The model under review builds one solid part; all positions refer to its coordinate system, in mm. A direction names the side the tool comes from. Round coordinates to 2 decimals unless told otherwise and drop trailing zeros. Loops run counter-clockwise (first coordinate to the right, second up) from the corner with the lowest first, then second, coordinate; pieces in that order, holes last. Notation, with made-up numbers: M 65,-32 L 83,-32 A15 cw 83,-9 Z; hole C 71,-15.75 d10. An arc over 180 degrees is marked long. Answer as a JSON object with one key per item and string values. Group by question number.
Item 1: To check wall thickness, follow line 1 (Z direction, x = -9, y = 0.3); line 2 (Z direction, x = -87.5, y = 3.35); line 3 (Z direction, x = 0, y = 4.6). State the ranges of each line that lie inside material, in increasing order.
Item 2: Insertion check: P1, Ø8, axis at x = -88.58, z = -718, coming from the +Y side; P2, Ø5.5, axis at x = -30.98, z = -734, coming from the -Y side; P3, Ø1, axis at y = 1, z = 82, coming from the +X side; P4, Ø3, axis at y = 3, z = 297.5, coming from the +X side. Each pin has a flat end and moves straight along its axis. Give the tip position at first contact, or say it passes through.
Item 3: The part is to be moulded in two halves that separate along Z. For faces 1 (the face through (-181, 0, 10)), 2 (the face through (85.906, 2.465, 451.968)), 3 (the face through (-249.98, 2.46, 10.62)), say which applies: +Z half, -Z half, draft (parallel to the pull), parting line (faces both ways), or undercut.
Item 4: Tool access review of faces 4 (the face through (84.55, 2.46, -443.41)), 5 (the face through (-149.945, 2.535, -4.063)): name each direction out of +Z, -Z, +X, -X, +Y, -Y from which nothing blocks a thin tool from reaching the whole face with its end or side.
Item 5: Consider section C-C (x = -105.5). Give the boundary of the cut face in (y, z).
Item 6: Consider section B-B (y = 1.8). State how many separate pieces and enclosed holes the cut face has, and give its area (3 significant figures).
Item 7: Consider section D-D (z = 0). Give the boundary of the cut face in (x, y), and give its area (3 significant figures).
Item 8: Consider section A-A (x = 0). Give the boundary of the cut face in (y, z).
Autodesk Inventor part; units mm, degrees
ref_plane "YZ Plane" through (0, 0, 0) normal (1, 0, 0) x (0, 1, 0)
ref_plane "XZ Plane" through (0, 0, 0) normal (0, 1, 0) x (-1, 0, 0)
ref_plane "XY Plane" through (0, 0, 0) normal (0, 0, 1) x (1, 0, 0)
sketch "Sketch1" plane through (0, 0, 0) normal (0, 1, 0) x (-1, 0, 0)
  arc A0 (0, -750) -> (0, 750) centre (-2762.5, 0) ccw construction
  line L0 (-22.4292, 0) -> (36.1533, 0) construction
  line L1 (0, 750) -> (0, -750) construction
  line L2 (150, 750) -> (-150, 750)
  line L3 (150, -750) -> (-150, -750)
  arc A1 (150, -750) -> (150, 750) centre (-2612.5, 0) ccw
  arc A2 (-150, -750) -> (-150, 750) centre (-2912.5, 0) ccw
  point P0 (0, 0)
  point P1 (100, 0)
  point P2 (250, 0)
  point P3 (-50, 0)
  dimension "d0" = 1500
  dimension "d1" = 100
  dimension "d2" = 300
  dimension "d3" = 150
  dimension "d4" = 150
extrude "Extrusion1" add sketch "Sketch1" along normal blind 5
sketch "Sketch2" plane through (0, 5, 0) normal (0, 1, 0) x (1, 0, 0)
  line L0 (-150, -750) -> (150, -750) construction
  arc A0 (150, 750) -> (150, -750) centre (2912.5, 0) ccw construction
  line L1 (150, 750) -> (-150, 750) construction
  arc A1 (-150, 750) -> (-150, -750) centre (2612.5, 0) ccw construction
  line L2 (-150, -750) -> (150, -750) construction
  arc A2 (150, 750) -> (150, -750) centre (2912.5, 0) ccw construction
  line L3 (150, -750) -> (150, -750) construction
  line L4 (150, -750) -> (150, -750) construction
  line L5 (150, 750) -> (-150, 750) construction
  line L6 (150, -750) -> (150, 750) construction
  circle A3 centre (0, 0) radius 150
  line L7 (150, 0) -> (-250, 0) construction
  arc A4 (-150, 750) -> (-150, -750) centre (2612.5, 0) ccw construction
  circle A5 centre (0, 0) radius 36 construction
  point P0 (-36, 0)
  point P1 (-18, -31.1769)
  point P2 (18, -31.1769)
  point P3 (36, 0)
  point P4 (18, 31.1769)
  point P5 (-18, 31.1769)
  dimension "d42" = 72
  dimension "d9" = 300
  dimension "d45" = 360
extrude "Extrusion2" cut sketch "Sketch2" against normal through all
sketch "Sketch3" plane through (0, 5, 0) normal (0, 1, 0) x (1, 0, 0)
  line L0 (-150, -750) -> (150, -750)
  arc A0 (53.4335, -140.1601) -> (150, -750) centre (2912.5, 0) ccw
  line L1 (150, 750) -> (-150, 750)
  arc A1 (-150, 750) -> (-150, -750) centre (2612.5, 0) ccw
  line L2 (-137.7375, -734) -> (129.1556, -734)
  arc A2 (129.1556, 734) -> (129.1556, -734) centre (2912.5, 0) ccw
  line L3 (129.1556, 734) -> (-137.7375, 734)
  arc A3 (-137.7375, 734) -> (-137.7375, -734) centre (2612.5, 0) ccw
  line L4 (-141.9579, -718) -> (124.9853, -718)
  arc A4 (53.4335, 140.1601) -> (53.4335, -140.1601) centre (0, 0) ccw
  arc A5 (150, 750) -> (53.4335, 140.1601) centre (2912.5, 0) ccw
  point P0 (0, 0)
  point P1 (-84.3589, -734)
  point P2 (-30.9803, -734)
  point P3 (22.3983, -734)
  point P4 (75.777, -734)
  point P5 (129.1556, -734)
  point P6 (-88.5793, -718)
  point P7 (-35.2007, -718)
  point P8 (18.1779, -718)
  point P9 (71.5566, -718)
  point P10 (124.9352, -718)
  dimension "d10" = 16
  dimension "d11" = 266.8931
  dimension "d14" = 53.3786
  dimension "d26" = 16
  dimension "d27" = 16
  dimension "d30" = 53.3786
hole "Hole2" at (-137.7375, 5, 734) at (-84.3589, 5, 734) at (-30.9803, 5, 734) at (22.3983, 5, 734) at (75.777, 5, 734) at (129.1556, 5, 734) at (-141.9579, 5, 718) at (-88.5793, 5, 718) at (-35.2007, 5, 718) at (18.1779, 5, 718) at (71.5566, 5, 718) at (124.9352, 5, 718) direction (0, -1, 0) diameter 6.2 end through all
mirror "Mirror1" about plane through (0, 0, 0) normal (0, 0, 1) of "Hole2"
equation "\"d27\" = d26"
properties part number "Floor"
Geometry results:
{
 "1": {"line 1": "z = -750 to -149.73, 149.73 to 750", "line 2": "z = -750 to -720.91, -715.09 to -121.83, 121.83 to 715.09, 720.91 to 750", "line 3": "z = -750 to -150, 150 to 750"},
 "2": {"P1": "stops at y = 5", "P2": "passes through", "P3": "stops at x = -125.27", "P4": "stops at x = 65.66"},
 "3": {"face 1": "draft", "face 2": "undercut", "face 3": "parting line"},
 "4": {"face 4": "+X, +Y, -Y", "face 5": "+Y, -Y"},
 "5": {"outline": "M 0,-750 L 5,-750 L 5,-106.63 L 0,-106.63 Z; M 0,106.63 L 5,106.63 L 5,750 L 0,750 Z"},
 "6": {"separate pieces": "1", "enclosed holes": "24", "area": "399,000 mm^2"},
 "7": {"outline": "M -250,0 L -150,0 L -150,5 L -250,5 Z", "area": "500 mm^2"},
 "8": {"outline": "M 0,-750 L 5,-750 L 5,-150 L 0,-150 Z; M 0,150 L 5,150 L 5,750 L 0,750 Z"}
}
